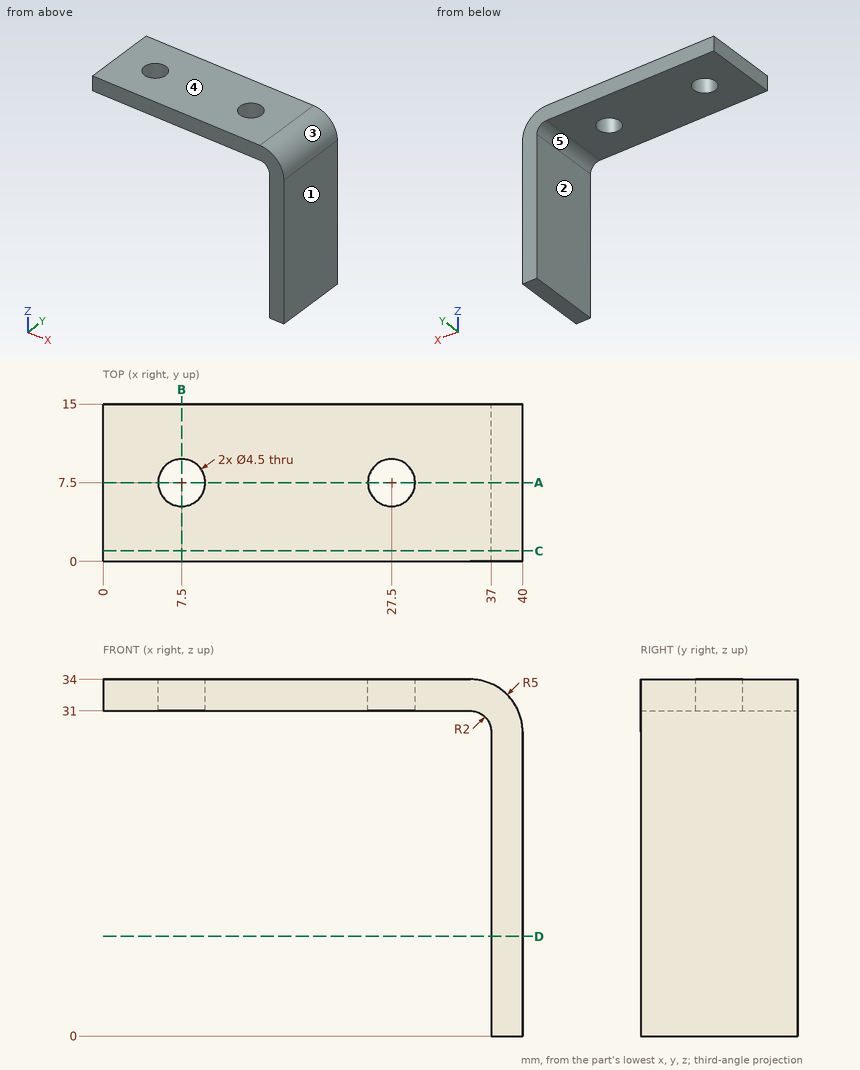
Geometry: see drawing. Coordinates: mm, zero at the bounding-box minimum. A direction names the side the tool comes from. Give positions to 0.01 mm unless a question says otherwise; leave off trailing zeros. Order: outer loops, then holes, each group sorted by start corner. A loop starts at its lowest first (then second) coordinate and runs counter-clockwise, first axis right, second up. Notation, with made-up numbers: (84, 58) -> (125, 58) arc R24 ccw to (125, 68) -> close; hole circle Ø2 at (27, 0.5). An arc over 180 degrees is marked (long way). Write item = value, one per line.
Q1. Material intervals for line 1 (Y direction, x = 7.5, z = 32.5); line 2 (X direction, y = 7.5, z = 32.8); line 3 (X direction, y = 7.5, z = 32.4), sorted ascending. Write a range as from..to.
Data:
line_1 = 0..5.25, 9.75..15
line_2 = 0..5.25, 9.75..25.25, 29.75..38.25
line_3 = 0..5.25, 9.75..25.25, 29.75..38.67
Q2. Pin query (flat end, axial travel): pin 1 (6 mm diameter, centred on x = 7.5, y = 7.5, fed in from -Z); pin 2 (4 mm diameter, centred on y = 10, z = 11, fed in from -X); pin 3 (8 mm diameter, centred on x = 32, y = 5, fed in from -Z). Return the tip coordinate at first contact, or that it passes through.
Data:
pin_1 = 31
pin_2 = 37
pin_3 = 30.73
Q3. Set-up query: the marked faces 1 and 2. Return all of +Z, -Z, +X, -X, +Y, -Y with unobstructed straight access to the full face (end or side cutting, diameter ignored); none if empty.
Data:
face_1 = +Z, -Z, +X, +Y, -Y
face_2 = -Z, -X, +Y, -Y
Q4. Cut plane A-A, the plane y = 7.5. Output: boundary loops of the cut face in (x, z).
Data:
outline = (0, 31) -> (5.25, 31) -> (5.25, 34) -> (0, 34) -> close; (9.75, 31) -> (25.25, 31) -> (25.25, 34) -> (9.75, 34) -> close; (29.75, 31) -> (35, 31) arc R2 cw to (37, 29) -> (37, 0) -> (40, 0) -> (40, 29) arc R5 ccw to (35, 34) -> (29.75, 34) -> close
Q5. Pull-direction query (X, two-part tool) for the marked faces 3, 4 and 5; classes: released by +X, released by -X, zero draft, split by the parting line, or undercut.
Data:
face_3 = released by +X
face_4 = zero draft
face_5 = released by -X
Q6. Cut plane D-D, the plane z = 9.5. Output: boundary loops of the cut face in (x, y), and give its area (3 significant figures).
Data:
outline = (37, 0) -> (40, 0) -> (40, 15) -> (37, 15) -> close
area = 45.0 mm^2
Q7. Cut plane C-C, the plane y = 1. Output: boundary loops of the cut face in (x, z).
Data:
outline = (0, 31) -> (35, 31) arc R2 cw to (37, 29) -> (37, 0) -> (40, 0) -> (40, 29) arc R5 ccw to (35, 34) -> (0, 34) -> close
Q8. Cut plane B-B, the plane x = 7.5. Output: boundary loops of the cut face in (y, z).
Data:
outline = (0, 31) -> (5.25, 31) -> (5.25, 34) -> (0, 34) -> close; (9.75, 31) -> (15, 31) -> (15, 34) -> (9.75, 34) -> close
